The model under review builds one solid part; all positions refer to its coordinate system, in mm. A direction names the side the tool comes from. Coordinates: 2 decimals unless noted, no trailing zeros. Loops run counter-clockwise (first coordinate to the right, second up) from the corner with the lowest first, then second, coordinate; pieces in that order, holes last. Notation, with made-up numbers: (88, 46) - (135, 46) arc R13 ccw to (135, 70) - close; hole circle Ø6 at (80.5, 15). An arc over 180 degrees is marked (long way). One line per item, written item: value. Start each with the question number.
1. To check wall thickness, follow line 1 (Z direction, x = 0, y = 3); line 2 (Z direction, x = 0, y = 41); line 3 (Y direction, x = 8, z = 14). State the ranges of each line that lie inside material, in increasing order.
2. For faces 4 (the face through (12, 38, 0)), 5 (the face through (0, 8, -8)), 6 (the face through (-23.977, 21.241, -1.055)), list the 3-axis set-ups (+Z, -Z, +X, -X, +Y, -Y) from which the entire face can be reached by the end or side of a thin tool; tool diameter is ignored.
3. Insertion check: P1, Ø8, axis at y = 22, z = -8.5, coming from the +X side; P2, Ø2.5, axis at x = 9, z = 0, coming from the -Y side; P3, Ø1, axis at y = 40, z = 7, coming from the +X side. Each pin has a flat end and moves straight along its axis. Give the tip position at first contact, or say it passes through.
4. Mouldability with a two-part tool opening along Z and no side actions: class faces 1 (the face through (-4.584, 0.146, 20.643)), 2 (the face through (0, 38, 13)), 3 (the face through (0, -19, 0)) as +Z half, -Z half, draft (parallel to the pull), parting line (faces both ways), or undercut.
5. We need section B-B, the plane y = 32. Give the boundary of the cut face in (x, z).
from build123d import *

# Parameters (mm, degrees)
SKETCH_1_R          = 24
EXTRUDE_1_DEPTH     = 46
SKETCH_3_R          = 6
EXTRUDE_2_DEPTH     = 2
CHAMFER_1_SIZE      = 6
CHAMFER_2_SIZE      = 3
SKETCH_4_R          = 1.5
CUT_EXTRUDE_1_DEPTH = 8
SKETCH_5_R          = 1.5
CUT_EXTRUDE_2_DEPTH = 8
SKETCH_6_R          = 2.5
EXTRUDE_3_DEPTH     = 19


with BuildPart() as part:
    # 草图1 → 凸台-拉伸1 (new body)
    with BuildSketch(Plane(origin=(0, 0, 0), x_dir=(1, 0, 0), z_dir=(0, 1, 0))):
        Circle(SKETCH_1_R)
    extrude(amount=EXTRUDE_1_DEPTH)

    # 草图3 → 凸台-拉伸2 (add)
    with BuildSketch(Plane(origin=(0, 46, 0), x_dir=(1, 0, 0), z_dir=(0, 1, 0))):
        Circle(SKETCH_3_R)
    extrude(amount=EXTRUDE_2_DEPTH)

    # 倒角1
    chamfer_1_edges = [part.edges().sort_by_distance(p)[0] for p in [
        (-24, 46, 0),
    ]]
    chamfer(chamfer_1_edges, length=CHAMFER_1_SIZE)

    # 倒角2
    chamfer_2_edges = [part.edges().sort_by_distance(p)[0] for p in [
        (-24, 0, 0),
    ]]
    chamfer(chamfer_2_edges, length=CHAMFER_2_SIZE)

    # 草图4 → 切除-拉伸1 (cut)
    with BuildSketch(Plane.XZ.offset(-46)):
        with Locations((0, 12.5)):
            Circle(SKETCH_4_R)
        with Locations((-12.5, 0)):
            Circle(SKETCH_4_R)
        with Locations((12.5, 0)):
            Circle(SKETCH_4_R)
        with Locations((0, -12.5)):
            Circle(SKETCH_4_R)
    extrude(amount=CUT_EXTRUDE_1_DEPTH, mode=Mode.SUBTRACT)

    # 草图5 → 切除-拉伸2 (cut)
    with BuildSketch(Plane.XZ):
        with Locations((0, 8.5)):
            Circle(SKETCH_5_R)
        with Locations((8.5, 0)):
            Circle(SKETCH_5_R)
        with Locations((0, -8.5)):
            Circle(SKETCH_5_R)
        with Locations((-8.5, 0)):
            Circle(SKETCH_5_R)
    extrude(amount=-CUT_EXTRUDE_2_DEPTH, mode=Mode.SUBTRACT)

    # 草图6 → 凸台-拉伸3 (add)
    with BuildSketch(Plane.XZ):
        Circle(SKETCH_6_R)
    extrude(amount=EXTRUDE_3_DEPTH)


solid = part.part
Findings below:
1. line 1: -24 to -10, -7 to 7, 10 to 24
1. line 2: -23 to -14, -11 to 11, 14 to 23
1. line 3: 0 to 46
2. face 4: +Y
2. face 5: -Y
2. face 6: +Y, -Y
3. P1: x = 23.57
3. P2: y = 0
3. P3: x = 23.1
4. face 1: parting line
4. face 2: undercut
4. face 3: draft
5. outline: circle Ø48 at (0, 0)
